from build123d import *

# Parameters (mm, degrees)
BOSS_EXTRUDE1_START = 12
BOSS_EXTRUDE1_DEPTH = 81.818884
SKETCH1_OUTSIDE_W   = 111.208
SKETCH1_OUTSIDE_H   = 107.499
CUT_EXTRUDE1_DEPTH  = 86.261649485
CUT_EXTRUDE2_START  = -37.210696
CUT_EXTRUDE2_DEPTH  = 27
SKETCH5_R           = 2
CUT_EXTRUDE4_DEPTH  = 85.8164494


with BuildPart() as part:
    # Sketch2 → Boss-Extrude1 (new body)
    with BuildSketch(Plane.XY.offset(BOSS_EXTRUDE1_START)):
        Polygon((-48.8453919, -1.977444406), (-7.943168155, -3), (-7.569819885, -2), (1.280407352, -2), (1.653755621, -3), (36.682523305, -2), (36.682523305, 0), (-48.8453919, 0), align=None)
    extrude(amount=-BOSS_EXTRUDE1_DEPTH)

    # Sketch1 outside → Cut-Extrude1 (cut, through all)
    with BuildSketch(Plane(origin=(0, 0, 0), x_dir=(1, 0, 0), z_dir=(0, 1, 0))):
        with Locations((-6.081, 28.9095)):
            Rectangle(SKETCH1_OUTSIDE_W, SKETCH1_OUTSIDE_H)
        with BuildLine():
            Line((-27.718637693, -3.492120904), (0, -12))
            Line((0, -12), (36.682523305, -6.114423246))
            Line((36.682523305, -6.114423246), (36.682523305, 54.145919103))
            Line((36.682523305, 54.145919103), (-10.674216271, 58))
            Line((-10.674216271, 58), (-26.6233986, 61.050643653))
            Line((-26.6233986, 61.050643653), (-47.053769098, 69.453098724))
            ThreePointArc((-47.053769098, 69.453098724), (-48.393579381, 68.911077159), (-47.880590401, 67.559884621))
            Line((-47.880590401, 67.559884621), (-27.718637693, 58.23156579))
            Line((-27.718637693, 58.23156579), (-10.674216271, 53))
            Line((-10.674216271, 53), (-10.674216271, 37.425437768))
            Line((-10.674216271, 37.425437768), (-26.6233986, 40.476081421))
            Line((-26.6233986, 40.476081421), (-47.053769098, 48.878536493))
            ThreePointArc((-47.053769098, 48.878536493), (-48.393579381, 48.336514928), (-47.880590401, 46.985322389))
            Line((-47.880590401, 46.985322389), (-27.718637693, 37.657003559))
            Line((-27.718637693, 37.657003559), (-10.674216271, 32.425437768))
            Line((-10.674216271, 32.425437768), (-10.674216271, 16.850875537))
            Line((-10.674216271, 16.850875537), (-26.6233986, 19.90151919))
            Line((-26.6233986, 19.90151919), (-47.053769098, 28.303974261))
            ThreePointArc((-47.053769098, 28.303974261), (-48.393579381, 27.761952696), (-47.880590401, 26.410760157))
            Line((-47.880590401, 26.410760157), (-27.718637693, 17.082441327))
            Line((-27.718637693, 17.082441327), (-10.674216271, 11.850875537))
            Line((-10.674216271, 11.850875537), (-10.674216271, -3.723686695))
            Line((-10.674216271, -3.723686695), (-26.6233986, -0.673043042))
            Line((-26.6233986, -0.673043042), (-47.053769098, 7.729412029))
            ThreePointArc((-47.053769098, 7.729412029), (-48.393579381, 7.187390465), (-47.880590401, 5.836197926))
            Line((-47.880590401, 5.836197926), (-27.718637693, -3.492120904))
        make_face(mode=Mode.SUBTRACT)
    extrude(amount=-CUT_EXTRUDE1_DEPTH, mode=Mode.SUBTRACT)

    # Sketch3 → Cut-Extrude2 (cut)
    with BuildSketch(Plane.XY.offset(CUT_EXTRUDE2_START)):
        Polygon((34.143841834, 0), (29.113394238, 0), (26.332255745, -2.295479066), (31.673105241, -2.143008687), align=None)
    extrude(amount=CUT_EXTRUDE2_DEPTH, mode=Mode.SUBTRACT)

    # Cut-Extrude3 cone 1 section (through the dimple's axis) → Cut-Extrude3 (revolve, cut)
    with BuildSketch(Plane(origin=(-2.644706267, 0, -27), x_dir=(0, 0, 1), z_dir=(1, 0, 0))):
        Polygon((0, 0), (2.9924, 0), (0, 3.442362422), align=None)
    revolve(axis=Axis((-2.644706267, 0, -27), (0, -1, 0)), mode=Mode.SUBTRACT)

    # Sketch5 → Cut-Extrude4 (cut, through all)
    with BuildSketch(Plane(origin=(0, 0, 0), x_dir=(1, 0, 0), z_dir=(0, 1, 0))):
        with Locations(Location((-2.644706267, 27, 0), (0, 0, 270))):
            Circle(SKETCH5_R)
    extrude(amount=-CUT_EXTRUDE4_DEPTH, mode=Mode.SUBTRACT)


solid = part.part
The model under review builds one solid part; all positions refer to its coordinate system, in mm. A direction names the side the tool comes from. Round coordinates to 2 decimals unless told otherwise and drop trailing zeros. Write each loop counter-clockwise with the first axis right and the second up, starting at its lowest first coordinate (ties: lowest second). Pieces come first, ordered by that corner, then holes. Notation, with made-up numbers: M -38.5,62.25 L -13.5,62.25 A18 cw -13.5,68.25 Z; hole C 85.5,41.5 d4. An arc over 180 degrees is marked long. Use a Markdown table: item, result. Add a question column.
Q1. We need section D-D, the plane x = 9. State the section outline as (y, z) points.
Q2. The part is to be moulded in two halves that separate along X. For faces 6 (the face through (-37.941, -1.235, -1.237)), 7 (the face through (13.336, -1.146, -56.046)), 8 (the face through (-18.537, -1.445, -18.355)), say which applies: pulls with the +X half, pulls with the -X half, needs draft (parallel to the pull), parting line crosses it, or undercut.
Q3. To check wall thickness, follow line 1 (Z direction, x = -14.5, y = -2.4); line 2 (Z direction, x = -16, y = -1.5) (3 decimals); line 3 (X direction, y = -1.55, z = -27). State the ranges of each line that lie inside material, in increasing order.
Q4. Machinability: for faces 1 (the face through (-19.3, -1.4, -14.5)), 2 (the face through (30, -1, -10.211)), 3 (the face through (-10.674, -1, -45)), 4 (the face through (-14.053, -1.479, 7.687)), 5 (the face through (-3, -2, -22)), which of the approach directions +Z, -Z, +X, -X, +Y, -Y give a long, thin tool a straight path to every point of the face, cutting with its end or side? Answer none if there is none.
Q5. We need section B-B, the plane x = -30. State the section outline as (y, z) points, plus the area to 3 significant figures.
Q6. We need section A-A, the plane z = -43.5. State the section outline as (x, y) points.
Q7. Insertion check: pin 1 (3 mm diameter, centred on x = -2.64, z = -27, fed in from +Y); pin 2 (1.5 mm diameter, centred on y = -1, z = -2.5, fed in from -X); pin 3 (0.9 mm diameter, centred on y = -2, z = -44, fed in from -X); pin 4 (1.5 mm diameter, centred on x = 7.5, z = -10.5, fed in from -Y). Each pin has a flat end and moves straight along its axis. Give the tip position at first contact, or say it passes through.
Q8. We need section C-C, the plane y = -0.6. Count the separate pieces of the cut face and the enclosed holes in it, plus the area to 3 significant figures.
Findings below:
| question | item | result |
|---|---|---|
| 1 | outline | M -2.79,-56.4 L 0,-56.4 L 0,10.56 L -2.79,10.56 Z |
| 2 | face 6 | pulls with the -X half |
| 2 | face 7 | pulls with the +X half |
| 2 | face 8 | undercut |
| 3 | line 1 | z = -58.73 to -54.17, -38.16 to -33.6, -17.58 to -13.03, 2.99 to 7.55 |
| 3 | line 2 | z = -59.019 to -54.635, -38.444 to -34.06, -17.87 to -13.486, 2.705 to 7.089 |
| 3 | line 3 | x = -48.42 to -43.88, -10.67 to -4.64, -0.64 to 27.24, 32.36 to 36.68 |
| 4 | face 1 | -X, +Y, -Y |
| 4 | face 2 | none |
| 4 | face 3 | +Y, -Y |
| 4 | face 4 | +Z, -X, +Y, -Y |
| 4 | face 5 | +Z, -Z, -Y |
| 5 | outline | M -2.45,-62.44 L 0,-62.44 L 0,-59.29 L -2.45,-59.29 Z; M -2.45,-41.86 L 0,-41.86 L 0,-38.71 L -2.45,-38.71 Z; M -2.45,-21.29 L 0,-21.29 L 0,-18.14 L -2.45,-18.14 Z; M -2.45,-0.72 L 0,-0.72 L 0,2.44 L -2.45,2.44 Z |
| 5 | area | 30.9 mm² |
| 6 | outline | M -40.35,-2.19 L -33.98,-2.35 L -33.98,0 L -40.35,0 Z; M -10.67,-2.93 L -7.94,-3 L -7.57,-2 L 1.28,-2 L 1.65,-3 L 36.68,-2 L 36.68,0 L -10.67,0 Z |
| 7 | pin 1 | passes through |
| 7 | pin 2 | stops at x = -42.29 |
| 7 | pin 3 | stops at x = -42.4 |
| 7 | pin 4 | stops at y = -2.85 |
| 8 | separate pieces | 1 |
| 8 | enclosed holes | 2 |
| 8 | area | 3,440 mm² |
